Autodesk Inventor part; units mm, degrees
ref_plane "YZ Plane" through (0, 0, 0) normal (1, 0, 0) x (0, 1, 0)
ref_plane "XZ Plane" through (0, 0, 0) normal (0, 1, 0) x (-1, 0, 0)
ref_plane "XY Plane" through (0, 0, 0) normal (0, 0, 1) x (1, 0, 0)
sketch "Sketch1" plane through (0, 0, 0) normal (0, 1, 0) x (-1, 0, 0)
  line L0 (22.5, -30) -> (-22.5, -30)
  line L1 (-22.5, -30) -> (-22.5, 30)
  line L2 (-22.5, 30) -> (22.5, 30)
  line L3 (22.5, 30) -> (22.5, -30)
  line L4 (0, 0) -> (0, -2.1911) construction
  line L5 (0, 0) -> (-2.34, 0) construction
  line L6 (15.5, -15.5) -> (-15.5, -15.5) construction
  line L7 (-15.5, -15.5) -> (-15.5, 15.5) construction
  line L8 (-15.5, 15.5) -> (15.5, 15.5) construction
  line L9 (15.5, 15.5) -> (15.5, -15.5) construction
  circle A0 centre (15.5, -15.5) radius 2.5
  circle A1 centre (-15.5, -15.5) radius 2.5
  circle A2 centre (-15.5, 15.5) radius 2.5
  circle A3 centre (15.5, 15.5) radius 2.5
  circle A4 centre (0, -25) radius 2.5
  circle A5 centre (0, 25) radius 2.5
  line L10 (0, -25) -> (0, -30) construction
  line L11 (0, 30) -> (0, 25) construction
  circle A6 centre (0, 0) radius 7.5
  point P0 (0, -1.0955)
  dimension "d6" = 60
  dimension "d7" = 45
  dimension "d8" = 31
  dimension "d9" = 5
  dimension "d10" = 5
  dimension "d11" = 5
  dimension "d12" = 5
  dimension "d13" = 5
  dimension "d14" = 5
  dimension "d15" = 15
extrude "Extrusion1" add sketch "Sketch1" along normal blind 8
properties part number "XMotorMount"
Can you work these out from the model? Positions are in its coordinate system, mm. Round coordinates to 2 decimals unless told otherwise and drop trailing zeros. Loops run counter-clockwise (first coordinate to the right, second up) from the corner with the lowest first, then second, coordinate; pieces in that order, holes last. Notation, with made-up numbers: (-28, 58.5) -> (24, 58.5) arc R34 ccw to (24, 91.5) -> close; hole circle Ø4 at (69.25, 36.25). An arc over 180 degrees is marked (long way). Answer in a Markdown table with one row per item.
Item 1: Suppose I cut it at C-C, the plane z = -15.5. List the corners of the cut face in (x, y) for me.
Answer block:
| item | result |
|---|---|
| outline | (-22.5, 0) -> (-18, 0) -> (-18, 8) -> (-22.5, 8) -> close; (-13, 0) -> (13, 0) -> (13, 8) -> (-13, 8) -> close; (18, 0) -> (22.5, 0) -> (22.5, 8) -> (18, 8) -> close |
Item 2: Will this pin go through, and if not, where does the flat tip stop? P1, Ø4, axis at x = 0, z = 25, coming from the +Y side.
Answer block:
| item | result |
|---|---|
| P1 | through |
Item 3: Suppose I cut it at D-D, the plane y = 2.75. List the corners of the cut face in (x, z) for me.
Answer block:
| item | result |
|---|---|
| outline | (-22.5, -30) -> (22.5, -30) -> (22.5, 30) -> (-22.5, 30) -> close; hole circle Ø5 at (-15.5, -15.5); hole circle Ø5 at (-15.5, 15.5); hole circle Ø15 at (0, 0); hole circle Ø5 at (0, -25); hole circle Ø5 at (0, 25); hole circle Ø5 at (15.5, -15.5); hole circle Ø5 at (15.5, 15.5) |
Item 4: We'd pull the mould along Z, two halves only. Please class faces 1 (the flat face through (0, 4, -30)), 2 (the flat face through (-5, 8, -6)), 3 (the cylindrical face through (0.33, 3.94, -27.48)): released by +Z, released by -Z, zero draft, split by the parting line, or undercut.
Answer block:
| item | result |
|---|---|
| face 1 | released by -Z |
| face 2 | zero draft |
| face 3 | undercut |
Item 5: Suppose I cut it at B-B, the plane x = 15.5. List the corners of the cut face in (y, z) for me.
Answer block:
| item | result |
|---|---|
| outline | (0, -30) -> (8, -30) -> (8, -18) -> (0, -18) -> close; (0, -13) -> (8, -13) -> (8, 13) -> (0, 13) -> close; (0, 18) -> (8, 18) -> (8, 30) -> (0, 30) -> close |
Item 6: Suppose I cut it at A-A, the plane z = 25. List the corners of the cut face in (x, y) for me.
Answer block:
| item | result |
|---|---|
| outline | (-22.5, 0) -> (-2.5, 0) -> (-2.5, 8) -> (-22.5, 8) -> close; (2.5, 0) -> (22.5, 0) -> (22.5, 8) -> (2.5, 8) -> close |
Item 7: If I drill on probe 1 along Z at (x, y) = (-15.5, 2.5); probe 2 along Z at (x, y) = (0, 3.5); probe 3 along Z at (x, y) = (-14, 2.5), over which ranges is the centre line in solid material (lowest first)?
Answer block:
| item | result |
|---|---|
| probe 1 | -30 to -18, -13 to 13, 18 to 30 |
| probe 2 | -30 to -27.5, -22.5 to -7.5, 7.5 to 22.5, 27.5 to 30 |
| probe 3 | -30 to -17.5, -13.5 to 13.5, 17.5 to 30 |
